```python
from build123d import *

# Parameters (mm, degrees)
BOSS_EXTRUDE1_DEPTH = 14
SKETCH2_R           = 2.5
CUT_EXTRUDE1_DEPTH  = 20
CUT_EXTRUDE2_REACH  = 22
SKETCH3_R           = 2


with BuildPart() as part:
    # Sketch1 → Boss-Extrude1 (new body)
    with BuildSketch(Plane(origin=(0, 0, 0), x_dir=(1, 0, 0), z_dir=(0, 1, 0))):
        Polygon((-10, -10), (10, -10), (10, 10), (-10, 10), (-10, 9), (9, 9), (9, -9), (-10, -9), align=None)
    extrude(amount=BOSS_EXTRUDE1_DEPTH)

    # Sketch2 → Cut-Extrude1 (cut)
    with BuildSketch(Plane.XY.offset(10)):
        with Locations((-4.081710117, 7)):
            Circle(SKETCH2_R)
    extrude(amount=-CUT_EXTRUDE1_DEPTH, mode=Mode.SUBTRACT)

    # Sketch3 → Cut-Extrude2 (cut, up to next)
    with BuildSketch(Plane(origin=(10, 0, 0), x_dir=(0, 0, -1), z_dir=(1, 0, 0)), mode=Mode.PRIVATE) as cut_extrude2_sk1:
        with Locations((0, 7)):
            Circle(SKETCH3_R)
    cut_extrude2_tool1 = extrude(cut_extrude2_sk1.sketch, amount=-CUT_EXTRUDE2_REACH, mode=Mode.PRIVATE) & part.part
    add(cut_extrude2_tool1.solids().sort_by_distance((10, 7, 0))[0], mode=Mode.SUBTRACT)


solid = part.part
```
Build history of the part. All positions in model axes, mm. A direction names the side the tool comes from. Give positions to 0.01 mm unless a question says otherwise; leave off trailing zeros. Loops run counter-clockwise (first coordinate to the right, second up) from the corner with the lowest first, then second, coordinate; pieces in that order, holes last.
Item 1: Slice it at B-B, the plane x = 0.5. List the corners of the cut face in (y, z).
Answers follow:
outline: (0, -10) - (14, -10) - (14, -9) - (0, -9) - close; (0, 9) - (14, 9) - (14, 10) - (0, 10) - close
Item 2: Slice it at A-A, the plane y = 7. List the corners of the cut face in (x, z), and give its area (3 significant figures).
Answers follow:
outline: (-10, -10) - (-6.58, -10) - (-6.58, -9) - (-10, -9) - close; (-10, 9) - (-6.58, 9) - (-6.58, 10) - (-10, 10) - close; (-1.58, -10) - (10, -10) - (10, -2) - (9, -2) - (9, -9) - (-1.58, -9) - close; (-1.58, 9) - (9, 9) - (9, 2) - (10, 2) - (10, 10) - (-1.58, 10) - close
area: 44.0 mm2
Item 3: Slice it at D-D, the plane x = -3.75. List the corners of the cut face in (y, z).
Answers follow:
outline: (0, -10) - (4.52, -10) - (4.52, -9) - (0, -9) - close; (0, 9) - (4.52, 9) - (4.52, 10) - (0, 10) - close; (9.48, -10) - (14, -10) - (14, -9) - (9.48, -9) - close; (9.48, 9) - (14, 9) - (14, 10) - (9.48, 10) - close
Item 4: Drill centre lines: line 1 (Z direction, x = 7.5, y = 2); line 2 (Y direction, x = 9.65, z = 0); line 3 (X direction, y = 7.75, z = -5). Where is each one in solid material? Low to high.
Answers follow:
line 1: z = -10 to -9, 9 to 10
line 2: y = 0 to 5, 9 to 14
line 3: x = 9 to 10
Item 5: Flat gauge pin, fed straight in: pin 1 (8 mm diameter, centred on y = 11, z = 2, fed in from -X). Where does the tip first touch, or does it go through?
Answers follow:
pin 1: stops at x = 9
Item 6: Slice it at C-C, the plane z = 0. List the corners of the cut face in (x, y), and give its area (3 significant figures).
Answers follow:
outline: (9, 0) - (10, 0) - (10, 5) - (9, 5) - close; (9, 9) - (10, 9) - (10, 14) - (9, 14) - close
area: 10.0 mm2
Item 7: Pull direction X, two halves, no side cores. Call faces 3 (the face through (-2.93, 4.78, 9.51)), 4 (the face through (9, 8, -2)), 5 (the face through (0, 7, -10)): released by +X, released by -X, zero draft, split by the parting line, or undercut.
Answers follow:
face 3: undercut
face 4: released by -X
face 5: zero draft
Item 8: Which spindle directions (+Z, -Z, +X, -X, +Y, -Y) get a long thin tool onto all of the face, cutting with end or side? Do faces 1 (the face through (-10, 6.9, -9.5)), 2 (the face through (0, 7, 9)). Say none if no direction does.
Answers follow:
face 1: +Z, -Z, -X, +Y, -Y
face 2: -X, +Y, -Y
